```python
from build123d import *

# Parameters (mm, degrees)
SKIZZE3_W                            = 100
SKIZZE3_H                            = 5
AUFSATZ_LINEAR_AUSTRAGEN1_DEPTH      = 15
AUFSATZ_LINEAR_AUSTRAGEN1_DEPTH_BACK = 15
SKIZZE8_R                            = 3
SCHNITT_LINEAR_AUSTRAGEN1_DEPTH      = 21
SKIZZE10_R                           = 2.4
SCHNITT_LINEAR_AUSTRAGEN2_DEPTH      = 21


with BuildPart() as part:
    # Skizze3 → Aufsatz-Linear austragen1 (new body, two sides)
    with BuildSketch(Plane.XY) as aufsatz_linear_austragen1_sk:
        with Locations((15, 18.5)):
            Rectangle(SKIZZE3_W, SKIZZE3_H)
    extrude(amount=AUFSATZ_LINEAR_AUSTRAGEN1_DEPTH)
    extrude(aufsatz_linear_austragen1_sk.sketch, amount=-AUFSATZ_LINEAR_AUSTRAGEN1_DEPTH_BACK)

    # Skizze8 → Schnitt-Linear austragen1 (cut)
    with BuildSketch(Plane(origin=(0, 0, 0), x_dir=(1, 0, 0), z_dir=(0, 1, 0))):
        with Locations((53, 7.5)):
            Circle(SKIZZE8_R)
        with Locations((53, -7.5)):
            Circle(SKIZZE8_R)
    extrude(amount=SCHNITT_LINEAR_AUSTRAGEN1_DEPTH, mode=Mode.SUBTRACT)

    # Skizze10 → Schnitt-Linear austragen2 (cut)
    with BuildSketch(Plane(origin=(0, 0, 0), x_dir=(1, 0, 0), z_dir=(0, 1, 0))):
        with Locations((-25, 7.5)):
            Circle(SKIZZE10_R)
        with Locations((-25, -7.5)):
            Circle(SKIZZE10_R)
    extrude(amount=SCHNITT_LINEAR_AUSTRAGEN2_DEPTH, mode=Mode.SUBTRACT)


solid = part.part
```
Here's how the part is built. I have some questions about the finished solid (model axes, mm). Give positions to 0.01 mm unless a question says otherwise; leave off trailing zeros. Write each loop counter-clockwise with the first axis right and the second up, starting at its lowest first coordinate (ties: lowest second). Pieces come first, ordered by that corner, then holes.
(1) Imagine slicing it at C-C, the plane x = -25. Write out the boundary of the cut face in (y, z), and give its area (3 significant figures).
Output values:
outline: (16, -15) - (21, -15) - (21, -9.9) - (16, -9.9) - close; (16, -5.1) - (21, -5.1) - (21, 5.1) - (16, 5.1) - close; (16, 9.9) - (21, 9.9) - (21, 15) - (16, 15) - close
area: 102 mm2
(2) Imagine slicing it at B-B, the plane y = 18.65. Write out the boundary of the cut face in (x, z).
Output values:
outline: (-35, -15) - (65, -15) - (65, 15) - (-35, 15) - close; hole circle Ø4.8 at (-25, -7.5); hole circle Ø4.8 at (-25, 7.5); hole circle Ø6 at (53, -7.5); hole circle Ø6 at (53, 7.5)
(3) Thinking about a two-plate mould opening in X: for faces 1 (the face through (14, 21, 0)), 2 (the face through (50, 18.5, 7.4)), 3 (the face through (-35, 18, 0)), which applies, pulls with the +X half, pulls with the -X half, needs draft (parallel to the pull), parting line crosses it, or undercut?
Output values:
face 1: needs draft
face 2: undercut
face 3: pulls with the -X half
(4) Imagine slicing it at A-A, the plane z = -7.5. Write out the boundary of the cut face in (x, y).
Output values:
outline: (-35, 16) - (-27.4, 16) - (-27.4, 21) - (-35, 21) - close; (-22.6, 16) - (50, 16) - (50, 21) - (-22.6, 21) - close; (56, 16) - (65, 16) - (65, 21) - (56, 21) - close
(5) If I drill on L1, parallel to Z at x = 53, y = 17.4; L2, parallel to X at y = 19.25, z = -7.5; L3, parallel to Z at x = -25, y = 17.25, over which ranges is the centre line in solid material (lowest first)?
Output values:
L1: z = -15 to -10.5, -4.5 to 4.5, 10.5 to 15
L2: x = -35 to -27.4, -22.6 to 50, 56 to 65
L3: z = -15 to -9.9, -5.1 to 5.1, 9.9 to 15
